Autodesk Inventor part; units mm, degrees
ref_plane "YZ Plane" through (0, 0, 0) normal (1, 0, 0) x (0, 1, 0)
ref_plane "XZ Plane" through (0, 0, 0) normal (0, 1, 0) x (-1, 0, 0)
ref_plane "XY Plane" through (0, 0, 0) normal (0, 0, 1) x (1, 0, 0)
ref_plane "Work Plane1" through (0, 0, 0) normal (0, 0, 1) x (1, 0, 0)
sketch "Sketch1" plane through (0, 0, 0) normal (0, 0, 1) x (1, 0, 0)
  circle A0 centre (5.5332, 19.4257) radius 2.45 construction
  circle A1 centre (-14.4668, 30.9727) radius 2.45 construction
  circle A2 centre (5.5332, 42.5198) radius 2.45 construction
  line L0 (12.5332, 12.4257) -> (-21.4668, 12.4257)
  line L1 (-21.4668, 12.4257) -> (-21.4668, 49.5198)
  line L2 (-21.4668, 49.5198) -> (12.5332, 49.5198)
  line L3 (12.5332, 49.5198) -> (12.5332, 12.4257)
  circle A3 centre (5.5332, 19.4257) radius 2.45
  circle A4 centre (-14.4668, 30.9727) radius 2.45
  circle A5 centre (5.5332, 42.5198) radius 2.45
  point P0 (0, 0)
  dimension "d0" = 7
  dimension "d1" = 7
  dimension "d2" = 7
  dimension "d3" = 7
  dimension "d4" = 4.9
  dimension "d5" = 4.9
  dimension "d6" = 4.9
extrude "Extrusion1" add sketch "Sketch1" along normal blind 4
sketch "Sketch2" plane through (0, 0, 4) normal (0, 0, 1) x (1, 0, 0)
  line L0 (12.5332, 49.5198) -> (-21.4668, 49.5198)
  line L1 (-21.4668, 49.5198) -> (-21.4668, 12.4257)
  line L2 (-21.4668, 12.4257) -> (12.5332, 12.4257)
  line L3 (12.5332, 12.4257) -> (12.5332, 49.5198)
  circle A0 centre (5.5332, 42.5198) radius 2.45
  circle A1 centre (-14.4668, 30.9727) radius 2.45
  circle A2 centre (5.5332, 19.4257) radius 2.45
  point P0 (0, 0)
extrude "Extrusion2" add sketch "Sketch2" along normal blind 2 contours L3 L2 L1 L0 | A0 | A1 | A2
sketch "Sketch3" plane through (-21.4668, 12.4257, 0) normal (-1, 0, 0) x (0, 0, 1)
  line L0 (0, 37.094) -> (0, 0)
  line L1 (0, 0) -> (6, 0)
  line L2 (6, 37.094) -> (6, 0)
  line L3 (0, 37.094) -> (6, 37.094)
  line L4 (0, 37.094) -> (6, 37.094)
  line L5 (6, 37.094) -> (15, 37.094)
  line L6 (15, 37.094) -> (15, 0)
  line L7 (15, 0) -> (6, 0)
  line L8 (6, 0) -> (6, 37.094)
  circle A0 centre (10.5, 18.8104) radius 1.5
  point P0 (0, -12.4257)
  dimension "d11" = 9
  dimension "d12" = 3
extrude "Extrusion3" add sketch "Sketch3" against normal blind 10 contours L5 L6 L7 L2
sketch "Sketch4" plane through (-21.4668, 12.4257, 0) normal (-1, 0, 0) x (0, 0, 1)
  line L0 (7.55, 24.4104) -> (13.45, 24.4104)
  line L1 (13.45, 14.3104) -> (7.55, 14.3104)
  line L2 (13.45, 24.4104) -> (7.55, 24.4104)
  line L3 (7.55, 24.4104) -> (7.55, 14.3104)
  line L4 (7.55, 14.3104) -> (13.45, 14.3104)
  line L5 (13.45, 14.3104) -> (13.45, 24.4104)
  line L6 (13.65, 24.6104) -> (7.35, 24.6104)
  line L7 (7.35, 24.6104) -> (7.35, 14.1104)
  line L8 (7.35, 14.1104) -> (13.65, 14.1104)
  line L9 (13.65, 14.1104) -> (13.65, 24.6104)
  point P0 (0, -12.4257)
  dimension "d15" = 0.2
extrude "Extrusion4" cut sketch "Sketch4" against normal blind 10 contours L0 L5 L1 L3 | L9 L8 L7 L6
sketch "Sketch5" plane through (-21.4668, 49.5198, 0) normal (0, 1, 0) x (1, 0, 0)
  line L0 (9.45, -4) -> (4.55, -4)
  line L1 (34, 0) -> (0, 0)
  line L2 (0, 0) -> (0, -15)
  line L3 (0, -15) -> (10, -15)
  line L4 (10, -6) -> (10, -15)
  line L5 (34, -6) -> (10, -6)
  line L6 (34, 0) -> (34, -6)
  circle A0 centre (5, -10.5) radius 1.4
  point P0 (21.4668, 0)
  point P1 (4.9, -8.2)
  dimension "d18" = 2.8
extrude "Extrusion5" cut sketch "Sketch5" against normal through all contours A0
sketch "Sketch6" plane through (0, 0, 6) normal (0, 0, 1) x (1, 0, 0)
  line L0 (-11.4668, 49.5198) -> (-11.4668, 12.4257)
  line L1 (-11.4668, 12.4257) -> (12.5332, 12.4257)
  line L2 (12.5332, 12.4257) -> (12.5332, 49.5198)
  line L3 (12.5332, 49.5198) -> (-11.4668, 49.5198)
  circle A0 centre (-14.4668, 30.9727) radius 2.45
  circle A1 centre (5.5332, 42.5198) radius 2.45
  circle A2 centre (5.5332, 33.4727) radius 1.4
  circle A3 centre (5.5332, 28.4727) radius 1.4
  point P0 (0, 0)
  dimension "d21" = 2.8
  dimension "d22" = 2.8
  dimension "d23" = 2.5
  dimension "d24" = 2.5
extrude "Extrusion6" cut sketch "Sketch6" along normal through all both and the other way through all contours A2 | A3
equation "\"d5\" = d4"
equation "\"d6\" = d4"
properties part number "30_cellSTORM_UC2_motorized_xystage_coupler_fibermount"
Check sheet for the modelled part. Datum: model origin and axes. Units: mm. A direction names the side the tool comes from. Round coordinates to 2 decimals unless told otherwise and drop trailing zeros. Order: outer loops, then holes, each group sorted by start corner. A loop starts at its lowest first (then second) coordinate and runs counter-clockwise, first axis right, second up.
Q1. Scan lines: L1, parallel to Y at x = 5.5, z = 2; L2, parallel to X at y = 18.5, z = 10.5; L3, parallel to Y at x = -18, z = 11. Record each from-to range of solid material in increasing order.
Filled sheet:
L1: y = 12.43 to 16.98, 21.88 to 27.07, 29.87 to 32.07, 34.87 to 40.07, 44.97 to 49.52
L2: x = -21.47 to -17.87, -15.07 to -11.47
L3: y = 12.43 to 26.54, 37.04 to 49.52
Q2. Set-up check for faces 5 (the face through (-17, 32, 7.35)), 6 (the face through (-1, 31, 6)), 7 (the face through (12.533, 31, 3)), 8 (the face through (-5, 49.52, 3)), 9 (the face through (-15, 31, 4)): record each of +Z, -Z, +X, -X, +Y, -Y from which the full face is reachable in a straight line by a thin tool's end or side.
Filled sheet:
face 5: +X, -X
face 6: +Z, +X, +Y, -Y
face 7: +Z, -Z, +X, +Y, -Y
face 8: +Z, -Z, +X, -X, +Y
face 9: -Z
Q3. Cross-section at C-C, the plane y = 43. Enter the section's corners in (x, z), plus the area to 3 significant figures.
Filled sheet:
outline: (-21.47, 0) - (3.13, 0) - (3.13, 4) - (7.94, 4) - (7.94, 0) - (12.53, 0) - (12.53, 6) - (-11.47, 6) - (-11.47, 15) - (-21.47, 15) - close; hole circle Ø2.8 at (-16.47, 10.5)
area: 269 mm2
Q4. Cross-section at A-A, the plane z = 10.5. Enter the section's corners in (x, y).
Filled sheet:
outline: (-21.47, 12.43) - (-17.87, 12.43) - (-17.87, 26.54) - (-21.47, 26.54) - close; (-21.47, 37.04) - (-17.87, 37.04) - (-17.87, 49.52) - (-21.47, 49.52) - close; (-15.07, 12.43) - (-11.47, 12.43) - (-11.47, 26.54) - (-15.07, 26.54) - close; (-15.07, 37.04) - (-11.47, 37.04) - (-11.47, 49.52) - (-15.07, 49.52) - close
Q5. Cross-section at B-B, the plane z = 8.25. Enter the section's corners in (x, y), plus the area to 3 significant figures.
Filled sheet:
outline: (-21.47, 12.43) - (-11.47, 12.43) - (-11.47, 26.54) - (-21.47, 26.54) - close; (-21.47, 37.04) - (-11.47, 37.04) - (-11.47, 49.52) - (-21.47, 49.52) - close
area: 266 mm2
Q6. Draft check along Z on faces 1 (the face through (6.18, 27.23, 3.04)), 2 (the face through (-5, 31, 0)), 3 (the face through (-17, 32, 13.65)), 4 (the face through (-17, 26.536, 9)). Enter one of: pulls with the +Z half, pulls with the -Z half, needs draft (parallel to the pull), parting line crosses it, or undercut.
Filled sheet:
face 1: needs draft
face 2: pulls with the -Z half
face 3: undercut
face 4: undercut
Q7. Depth check by flat-ended pin: P1, Ø2.5, axis at x = -16.47, z = 10.5, coming from the +Y side; P2, Ø10, axis at x = 1, y = 38.5, coming from the +Z side. Enter the tip coordinate at first touch or a pass-through.
Filled sheet:
P1: passes through
P2: stops at z = 6
Q8. Cross-section at D-D, the plane x = 7.5. Enter the section's corners in (y, z).
Filled sheet:
outline: (12.43, 0) - (17.96, 0) - (17.96, 4) - (20.89, 4) - (20.89, 0) - (41.06, 0) - (41.06, 4) - (43.98, 4) - (43.98, 0) - (49.52, 0) - (49.52, 6) - (12.43, 6) - close
